from build123d import *

# Parameters (mm, degrees)
EXTRUDE_1_DEPTH = 5
EXTRUDE_2_DEPTH = 5


with BuildPart() as part:
    # 草图1 → 凸台-拉伸1 (new body)
    with BuildSketch(Plane(origin=(0, 0, 0), x_dir=(1, 0, 0), z_dir=(0, 1, 0))):
        Polygon((-241.5, 0), (241.5, 0), (241.5, -225), (107, -404.5), (-107, -404.5), (-241.5, -225), align=None)
    extrude(amount=EXTRUDE_1_DEPTH)

    # 草图2 → 凸台-拉伸2 (add)
    with BuildSketch(Plane(origin=(0, 5, 0), x_dir=(1, 0, 0), z_dir=(0, 1, 0))):
        Polygon((-234.75, -6.5), (234.75, -6.5), (234.75, -221.833333333), (103, -397.5), (-103, -397.5), (-234.75, -221.833333333), align=None)
    extrude(amount=EXTRUDE_2_DEPTH)


solid = part.part
The model under review builds one solid part; all positions refer to its coordinate system, in mm. A direction names the side the tool comes from. Give positions to 0.01 mm unless a question says otherwise; leave off trailing zeros. Write each loop counter-clockwise with the first axis right and the second up, starting at its lowest first coordinate (ties: lowest second). Pieces come first, ordered by that corner, then holes. Notation, with made-up numbers: M 16,52 L 32,52 A31 ccw 32,89 Z; hole C 26.5,33.5 d4. An arc over 180 degrees is marked long. One line per question, with ' | ' between items. Start each with the question number.
Item 1: Wall thickness on line 1 (X direction, y = 8.5, z = 215.5); line 2 (Z direction, x = -65.5, y = 7); line 3 (Z direction, x = 182, y = 1.25): over which ranges is each line inside the solid? List them lowest first. Write a range as from..to.
Item 2: We need section B-B on x = 5. Write out the cut boundary in (y, z), plus the area to 3 significant figures.
Item 3: For faces 1 (the flat face through (-167.95, 7.46, 310.9)), 2 (the flat face through (169.797, 7.465, 308.437)), 3 (the flat face through (-173.309, 2.465, 316.006)), list the 3-axis set-ups (+Z, -Z, +X, -X, +Y, -Y) from which the entire face can be reached by the end or side of a thin tool; tool diameter is ignored.
Item 4: We need section A-A on y = 8.5. Write out the cut boundary in (x, z), plus the area to 3 significant figures.
Item 5: For pin 1 (5.5 mm diameter, centred on x = -51, y = 7.5, fed in from -Z); pin 2 (6 mm diameter, centred on y = 3.5, z = 363, fed in from -X); pin 3 (4 mm diameter, centred on y = 8, z = 104, fed in from +X); pin 4 (2 mm diameter, centred on y = 7.5, z = 308, fed in from +X) (3 decimals), all flat-tipped, find the tip position at first contact; note any pin that passes through.
Item 6: We need section C-C on z = 240. Write out the cut boundary in (x, y) (3 decimals).
Results found:
1) line 1: x = -234.75..234.75 | line 2: z = 6.5..397.5 | line 3: z = 0..304.41
2) outline: M 0,0 L 5,0 L 5,6.5 L 10,6.5 L 10,397.5 L 5,397.5 L 5,404.5 L 0,404.5 Z | area: 3,980 mm2
3) face 1: +Z, -X, +Y | face 2: +Z, +X, +Y | face 3: +Z, -X, +Y, -Y
4) outline: M -234.75,6.5 L 234.75,6.5 L 234.75,221.83 L 103,397.5 L -103,397.5 L -234.75,221.83 Z | area: 160,000 mm2
5) pin 1: stops at z = 0 | pin 2: stops at x = -140.34 | pin 3: stops at x = 234.75 | pin 4: stops at x = 170.875
6) outline: M -230.26,0 L 230.26,0 L 230.26,5 L 221.125,5 L 221.125,10 L -221.125,10 L -221.125,5 L -230.26,5 Z
